```python
from build123d import *

# Parameters (mm, degrees)
SKETCH_W        = 75
SKETCH_H        = 90
PAD_DEPTH       = 45
THICKNESS_T     = 5
SKETCH002_W     = 15
SKETCH002_H     = 90
POCKET_DEPTH    = 3.5
SKETCH003_W     = 79
SKETCH003_H     = 10
POCKET001_DEPTH = 5
SKETCH004_W     = 79
SKETCH004_H     = 10
POCKET002_DEPTH = 5
SKETCH005_W     = 79
SKETCH005_H     = 7
POCKET003_DEPTH = 90
SKETCH006_W     = 15
SKETCH006_H     = 15
SKETCH006_W_2   = 20
POCKET004_DEPTH = 5
SKETCH007_W     = 15
SKETCH007_H     = 15
SKETCH007_W_2   = 20
POCKET005_DEPTH = 5
SKETCH008_W     = 30
SKETCH008_H     = 15
POCKET006_DEPTH = 5
SKETCH009_W     = 30
SKETCH009_H     = 15
POCKET007_DEPTH = 5


with BuildPart() as part:
    # Sketch → Pad (new body)
    with BuildSketch(Plane.XY):
        Rectangle(SKETCH_W, SKETCH_H)
    extrude(amount=PAD_DEPTH)

    # Thickness
    thickness_openings = [part.faces().sort_by_distance(p)[0] for p in [
        (0, 0, 45),
    ]]
    offset(amount=THICKNESS_T, openings=thickness_openings, kind=Kind.INTERSECTION)

    # Sketch002 (on Face5 of Thickness) → Pocket (cut)
    with BuildSketch(Plane.XY):
        with Locations((30, 0)):
            Rectangle(SKETCH002_W, SKETCH002_H)
    extrude(amount=-POCKET_DEPTH, mode=Mode.SUBTRACT)

    # Sketch003 (on Face13 of Pocket) → Pocket001 (cut)
    with BuildSketch(Plane.XZ.offset(50)):
        with Locations((0, 40)):
            Rectangle(SKETCH003_W, SKETCH003_H)
    extrude(amount=-POCKET001_DEPTH, mode=Mode.SUBTRACT)

    # Sketch004 (on Face19 of Pocket001) → Pocket002 (cut)
    with BuildSketch(Plane(origin=(0, 50, 0), x_dir=(-1, 0, 0), z_dir=(0, 1, 0))):
        with Locations((0, 40)):
            Rectangle(SKETCH004_W, SKETCH004_H)
    extrude(amount=-POCKET002_DEPTH, mode=Mode.SUBTRACT)

    # Sketch005 (on Face12 of Pocket002) → Pocket003 (cut)
    with BuildSketch(Plane(origin=(0, 45, 0), x_dir=(-1, 0, 0), z_dir=(0, 1, 0))):
        with Locations((0, 38.5)):
            Rectangle(SKETCH005_W, SKETCH005_H)
    extrude(amount=-POCKET003_DEPTH, mode=Mode.SUBTRACT)

    # Sketch006 (on Face24 of Pocket003) → Pocket004 (cut)
    with BuildSketch(Plane(origin=(-42.5, 0, 0), x_dir=(0, -1, 0), z_dir=(-1, 0, 0))):
        with Locations((-27.5, 22.5)):
            Rectangle(SKETCH006_W, SKETCH006_H)
        with Locations((27.5, 22.5)):
            Rectangle(SKETCH006_W, SKETCH006_H)
        with Locations((0, 22.5)):
            Rectangle(SKETCH006_W_2, SKETCH006_H)
    extrude(amount=-POCKET004_DEPTH, mode=Mode.SUBTRACT)

    # Sketch007 (on Face38 of Pocket004) → Pocket005 (cut)
    with BuildSketch(Plane.YZ.offset(42.5)):
        with Locations((-27.5, 22.5)):
            Rectangle(SKETCH007_W, SKETCH007_H)
        with Locations((27.5, 22.5)):
            Rectangle(SKETCH007_W, SKETCH007_H)
        with Locations((0, 22.5)):
            Rectangle(SKETCH007_W_2, SKETCH007_H)
    extrude(amount=-POCKET005_DEPTH, mode=Mode.SUBTRACT)

    # Sketch008 (on Face26 of Pocket005) → Pocket006 (cut)
    with BuildSketch(Plane.XZ.offset(50)):
        with Locations((0, 17.5)):
            Rectangle(SKETCH008_W, SKETCH008_H)
    extrude(amount=-POCKET006_DEPTH, mode=Mode.SUBTRACT)

    # Sketch009 (on Face57 of Pocket006) → Pocket007 (cut)
    with BuildSketch(Plane(origin=(0, 50, 0), x_dir=(-1, 0, 0), z_dir=(0, 1, 0))):
        with Locations((0, 17.5)):
            Rectangle(SKETCH009_W, SKETCH009_H)
    extrude(amount=-POCKET007_DEPTH, mode=Mode.SUBTRACT)


solid = part.part
```
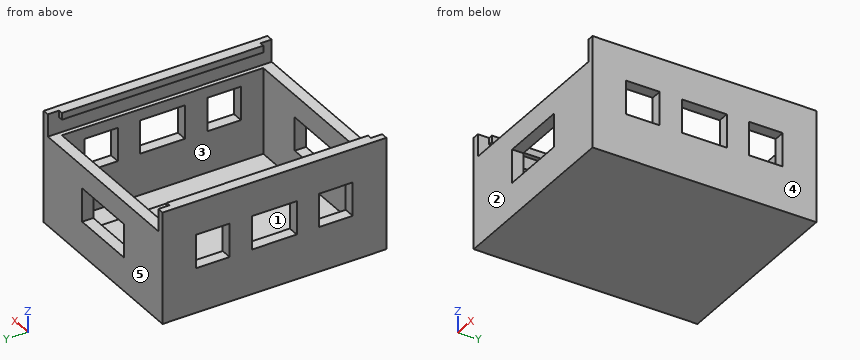
Here's how the part is built. I have some questions about the finished solid (model axes, mm). Face numbers are marked on the shaded views. A direction names the side the tool comes from. Give positions to 0.01 mm unless a question says otherwise; leave off trailing zeros. Write each loop counter-clockwise with the first axis right and the second up, starting at its lowest first coordinate (ties: lowest second). Pieces come first, ordered by that corner, then holes. Notation, with made-up numbers: (63, -5) -> (75, -5) arc R16 ccw to (75, 6) -> close; hole circle Ø2 at (-37.5, 14). An arc over 180 degrees is marked (long way). Write each question's results on one line, items separated by ' | '.
Item 1: Suppose I cut it at A-A on x = 7. Write out the boundary of the cut face in (y, z), plus the area to 3 significant figures.
Output:
outline: (-50, -5) -> (50, -5) -> (50, 10) -> (45, 10) -> (45, 0) -> (-45, 0) -> (-45, 10) -> (-50, 10) -> close; (-50, 25) -> (-45, 25) -> (-45, 35) -> (-50, 35) -> close; (45, 25) -> (50, 25) -> (50, 35) -> (45, 35) -> close | area: 700 mm^2
Item 2: For pin 1 Ø4 at (x, y) = (-3.5, -48) entering from +Z; pin 2 Ø5 at (x, y) = (32, 32.5) entering from +Z, each with a flat end and sliding along its axis, tell me the tip position at first contact or that it passes through.
Output:
pin 1: stops at z = 35 | pin 2: stops at z = -3.5
Item 3: Suppose I cut it at B-B on z = 13. Write out the boundary of the cut face in (x, y), plus the area to 3 significant figures.
Output:
outline: (-42.5, -50) -> (-15, -50) -> (-15, -45) -> (-37.5, -45) -> (-37.5, 45) -> (-15, 45) -> (-15, 50) -> (-42.5, 50) -> close; (15, -50) -> (42.5, -50) -> (42.5, 50) -> (15, 50) -> (15, 45) -> (37.5, 45) -> (37.5, -45) -> (15, -45) -> close | area: 1,450 mm^2
Item 4: Suppose I cut it at D-D on z = 7.5. Write out the boundary of the cut face in (x, y), plus the area to 3 significant figures.
Output:
outline: (-42.5, -50) -> (42.5, -50) -> (42.5, 50) -> (-42.5, 50) -> close; hole (-37.5, -45) -> (37.5, -45) -> (37.5, 45) -> (-37.5, 45) -> close | area: 1,750 mm^2
Item 5: If I drill on L1, parallel to X at y = 44.5, z = -0.5; L2, parallel to X at y = 31, z = 11.5; L3, parallel to Y at x = 9, z = 2, over which ranges is the centre line in solid material (lowest first)?
Output:
L1: x = -42.5 to 22.5, 37.5 to 42.5 | L2: x = -42.5 to -37.5, 37.5 to 42.5 | L3: y = -50 to -45, 45 to 50
Item 6: Suppose I cut it at C-C on y = -13. Write out the boundary of the cut face in (x, z).
Output:
outline: (-42.5, -5) -> (42.5, -5) -> (42.5, 45) -> (37.5, 45) -> (37.5, 42) -> (39.5, 42) -> (39.5, 35) -> (37.5, 35) -> (37.5, -3.5) -> (22.5, -3.5) -> (22.5, 0) -> (-37.5, 0) -> (-37.5, 35) -> (-39.5, 35) -> (-39.5, 42) -> (-37.5, 42) -> (-37.5, 45) -> (-42.5, 45) -> close
Item 7: We'd pull the mould along Y, two halves only. Please class the marked faces 3, 4 and 5: pulls with the +Y half, pulls with the -Y half, needs draft (parallel to the pull), parting line crosses it, or undercut.
Output:
face 3: undercut | face 4: needs draft | face 5: pulls with the +Y half
Item 8: On a 3-axis mill with a long thin cutter (end or side, diameter ignored), from which of +Z, -Z, +X, -X, +Y, -Y can I reach the whole of each face in a straight line? I mean the marked faces 1 and 2. Say none if no direction works.
Output:
face 1: +Z | face 2: +Z, -Z, +X, -X, -Y
